```python
from build123d import *

# Parameters (mm, degrees)
F0_W     = 72
F0_H     = 70
F1_DEPTH = 1
F2_W     = 5
F2_H     = 70
F3_DEPTH = 17
F4_R     = 1
F5_DEPTH = 5
F2_H_2   = 2
F6_DEPTH = 13
F7_R     = 0.5
F8_DEPTH = 70.001


with BuildPart() as f1:
    # F0 (on Top) → F1 (new body)
    with BuildSketch(Plane.XY):
        with Locations((-4, -15)):
            Rectangle(F0_W, F0_H)
    extrude(amount=F1_DEPTH)

    # F2 (on face) → F3 (join)
    with BuildSketch(Plane.XY.offset(1)):
        with Locations((-37.5, -15)):
            Rectangle(F2_W, F2_H)
    extrude(amount=F3_DEPTH)

    # F4 (on face) → F5 (cut, through all)
    with BuildSketch(Plane(origin=(-40, 0, 0), x_dir=(0, -1, 0), z_dir=(-1, 0, 0))):
        with Locations((-15, 9)):
            Circle(F4_R)
        with Locations((45, 9)):
            Circle(F4_R)
    extrude(amount=-F5_DEPTH, mode=Mode.SUBTRACT)

    # F2 (on face) → F6 (join)
    with BuildSketch(Plane.XY.offset(1)):
        with Locations((-0.6, 19)):
            Rectangle(F2_W, F2_H_2)
        with Locations((29.5, 19)):
            Rectangle(F2_W, F2_H_2)
        with Locations((-0.6, -49)):
            Rectangle(F2_W, F2_H_2)
        with Locations((29.5, -49)):
            Rectangle(F2_W, F2_H_2)
    extrude(amount=F6_DEPTH)

    # F7 (on face) → F8 (cut, through all)
    with BuildSketch(Plane.XZ.offset(50)):
        with Locations((-0.1, 7.5)):
            Circle(F7_R)
        with Locations((29, 7.5)):
            Circle(F7_R)
    extrude(amount=-F8_DEPTH, mode=Mode.SUBTRACT)


solid = f1.part
```
Check sheet for the modelled part. Datum: model origin and axes. Units: mm. A direction names the side the tool comes from. Give positions to 0.01 mm unless a question says otherwise; leave off trailing zeros. Order: outer loops, then holes, each group sorted by start corner. A loop starts at its lowest first (then second) coordinate and runs counter-clockwise, first axis right, second up. Notation, with made-up numbers: M -37,55.25 L -26,55.25 A29 ccw -26,93.25 Z; hole C 24.25,1 d10. An arc over 180 degrees is marked long. Answer in a Markdown table with one row per item.
1) Gauge pin test, flat ends, axial feed: P1, Ø3, axis at y = 10, z = 13, coming from the +X side; P2, Ø0.6, axis at x = -0.5, y = 19, coming from the +Z side; P3, Ø3, axis at x = 18, y = -41.5, coming from the +Z side. Record the tip position at first contact, or that the pin passes through.
Filled sheet:
| item | result |
|---|---|
| P1 | stops at x = -35 |
| P2 | stops at z = 14 |
| P3 | stops at z = 1 |
2) Cross-section at B-B, the plane z = 9. Enter the section's corners in (x, y), plus the area to 3 significant figures.
Filled sheet:
| item | result |
|---|---|
| outline | M -40,-50 L -35,-50 L -35,-46 L -40,-46 Z; M -40,-44 L -35,-44 L -35,14 L -40,14 Z; M -40,16 L -35,16 L -35,20 L -40,20 Z; M -3.1,-50 L 1.9,-50 L 1.9,-48 L -3.1,-48 Z; M -3.1,18 L 1.9,18 L 1.9,20 L -3.1,20 Z; M 27,-50 L 32,-50 L 32,-48 L 27,-48 Z; M 27,18 L 32,18 L 32,20 L 27,20 Z |
| area | 370 mm2 |
3) Thickness scan on L1, parallel to Z at x = 29, y = -49.55; L2, parallel to Y at x = -3, z = 8.5; L3, parallel to X at y = -17, z = 8.75. Record the ranges inside material, lowest first. Write a range as [from, to].
Filled sheet:
| item | result |
|---|---|
| L1 | z = [0, 7], [8, 14] |
| L2 | y = [-50, -48], [18, 20] |
| L3 | x = [-40, -35] |
4) Cross-section at A-A, the plane y = 15. Enter the section's corners in (x, z), plus the area to 3 significant figures.
Filled sheet:
| item | result |
|---|---|
| outline | M -40,0 L 32,0 L 32,1 L -35,1 L -35,8 L -40,8 Z; M -40,10 L -35,10 L -35,18 L -40,18 Z |
| area | 147 mm2 |
5) Release check for a two-part mould opening along Y. For faces 4 (the flat face through (-2, 20, 6)), 5 (the cylindrical face through (-38, 14, 9)), 6 (the flat face through (-38, -15, 18)) record: +Y half, -Y half, draft (parallel to the pull), parting line (faces both ways), or undercut.
Filled sheet:
| item | result |
|---|---|
| face 4 | +Y half |
| face 5 | undercut |
| face 6 | draft |
6) Access from +Z, -Z, +X, -X, +Y, -Y to the whole of each face (thin tool, end or side, straight path). Record for faces 1 (the flat face through (29, 19, 14)), 2 (the flat face through (27, 19, 7)), 3 (the flat face through (-1, 18, 7)).
Filled sheet:
| item | result |
|---|---|
| face 1 | +Z, +X, +Y, -Y |
| face 2 | +Z, +Y, -Y |
| face 3 | +Z, +X |
7) Cross-section at C-C, the plane x = -4. Enter the section's corners in (y, z).
Filled sheet:
| item | result |
|---|---|
| outline | M -50,0 L 20,0 L 20,1 L -50,1 Z |
